from build123d import *

# Parameters (mm, degrees)
SKETCH_1_R           = 1.5
EXTRUDE_1_DEPTH      = 2.5
EXTRUDE_2_DEPTH      = 7
EXTRUDE_2_DEPTH_BACK = 2.5
SKETCH_2_R           = 1.45
SKETCH_2_W           = 22.5
SKETCH_2_H           = 12
SKETCH_3_W           = 8
SKETCH_3_H           = 20
SKETCH_3_R           = 1.5
EXTRUDE_3_DEPTH      = 3
SKETCH_4_R           = 1.5
CUT_EXTRUDE_1_DEPTH  = 54.969899018
SKETCH_6_R           = 3.49128416
EXTRUDE_4_DEPTH      = 2.5
SKETCH_7_R           = 6
CUT_EXTRUDE_3_DEPTH  = 1.5
CUT_EXTRUDE_4_DEPTH  = 1.5
SKETCH_9_R           = 2.5
CUT_EXTRUDE_5_DEPTH  = 1.5
CUT_EXTRUDE_6_DEPTH  = 55.522930956
CHAMFER_1_SIZE       = 2
SKETCH_11_R          = 1.5
CUT_EXTRUDE_8_DEPTH  = 52.232314022
EXTRUDE_START        = -3
EXTRUDE_7_DEPTH      = 3
SKETCH_18_W          = 3
SKETCH_18_H          = 6.085719459
EXTRUDE_9_DEPTH      = 45
SKETCH_19_R          = 1.410967792
SKETCH_19_R_2        = 1.436695047
CUT_EXTRUDE_9_DEPTH  = 45
EXTRUDE_10_DEPTH     = 17.5
SKETCH_21_R          = 1.436695047
SKETCH_21_R_2        = 1.410967792
CUT_EXTRUDE_10_DEPTH = 17.5


with BuildPart() as part:
    # 草图1 → 凸台-拉伸1 (new body)
    with BuildSketch(Plane.XY):
        Polygon((4, 0), (0, 4), (0, 12), (-10, 17), (-10, 27), (45.5, 27), (45.5, 17), (35.5, 12), (35.5, 4), (31.5, 0), align=None)
        with Locations((4, 4)):
            Circle(SKETCH_1_R, mode=Mode.SUBTRACT)
        with Locations((31.5, 4)):
            Circle(SKETCH_1_R, mode=Mode.SUBTRACT)
        with Locations((7, 21)):
            Circle(SKETCH_1_R, mode=Mode.SUBTRACT)
        with Locations((28.5, 21)):
            Circle(SKETCH_1_R, mode=Mode.SUBTRACT)
    extrude(amount=EXTRUDE_1_DEPTH)

    # 草图2 → 凸台-拉伸2 (add, two sides: drawn at the far end of the back side and taken through both)
    with BuildSketch(Plane(origin=(0, 0, 0), x_dir=(-1, 0, 0), z_dir=(0, 0, -1)).offset(-EXTRUDE_2_DEPTH_BACK)):
        with BuildLine():
            Line((-35.2, 28.5), (-9.7, 28.5))
            Line((-9.7, 28.5), (-9.7, 23))
            Line((-9.7, 23), (-8.2, 23))
            Line((-8.2, 23), (-8.2, 22.240967365))
            ThreePointArc((-8.2, 22.240967365), (-10.4, 21), (-8.2, 19.759032635))
            Line((-8.2, 19.759032635), (-8.2, 19))
            Line((-8.2, 19), (-9.7, 19))
            Line((-9.7, 19), (-9.7, 13.5))
            Line((-9.7, 13.5), (-35.2, 13.5))
            Line((-35.2, 13.5), (-35.2, 19))
            Line((-35.2, 19), (-38.2, 19))
            Line((-38.2, 19), (-38.2, 23))
            Line((-38.2, 23), (-35.2, 23))
            Line((-35.2, 23), (-35.2, 28.5))
        make_face()
        with Locations((-35.95, 21)):
            Circle(SKETCH_2_R, mode=Mode.SUBTRACT)
        with Locations((-22.45, 21)):
            Rectangle(SKETCH_2_W, SKETCH_2_H, mode=Mode.SUBTRACT)
    extrude(amount=EXTRUDE_2_DEPTH + EXTRUDE_2_DEPTH_BACK)

    # 草图3 → 凸台-拉伸3 (add)
    with BuildSketch(Plane(origin=(0, 0, 0), x_dir=(-1, 0, 0), z_dir=(0, 0, -1))):
        with Locations((-4, 17)):
            Rectangle(SKETCH_3_W, SKETCH_3_H)
        with Locations((-2.5, 9.5)):
            Circle(SKETCH_3_R, mode=Mode.SUBTRACT)
        with Locations((-2.5, 18.5)):
            Circle(SKETCH_3_R, mode=Mode.SUBTRACT)
    extrude(amount=EXTRUDE_3_DEPTH)

    # 草图4 → 切除-拉伸1 (cut, through all)
    with BuildSketch(Plane(origin=(0, 0, -3), x_dir=(-1, 0, 0), z_dir=(0, 0, -1))):
        with Locations((-2.5, 9.5)):
            Circle(SKETCH_4_R)
        with Locations(Location((-7, 21, 0), (0, 0, 228.189685104))):
            Circle(SKETCH_4_R)
    extrude(amount=-CUT_EXTRUDE_1_DEPTH, mode=Mode.SUBTRACT)

    # 草图6 → 凸台-拉伸4 (add)
    with BuildSketch(Plane(origin=(0, 0, 0), x_dir=(-1, 0, 0), z_dir=(0, 0, -1))):
        with Locations((-27, 21)):
            Circle(SKETCH_6_R)
    extrude(amount=-EXTRUDE_4_DEPTH)

    # 草图7 → 切除-拉伸3 (cut)
    with BuildSketch(Plane(origin=(0, 0, 0), x_dir=(-1, 0, 0), z_dir=(0, 0, -1))):
        with Locations((-27.7, 21)):
            Circle(SKETCH_7_R)
    extrude(amount=-CUT_EXTRUDE_3_DEPTH, mode=Mode.SUBTRACT)

    # 草图8 → 切除-拉伸4 (cut)
    with BuildSketch(Plane(origin=(0, 0, 0), x_dir=(-1, 0, 0), z_dir=(0, 0, -1))):
        with BuildLine():
            ThreePointArc((-21.71878059, 17.962224138), (-18.800764933, 20.795559838), (-21.585591732, 23.759905678))
            ThreePointArc((-21.585591732, 23.759905678), (-22.24975442, 23.944667862), (-22.761132033, 24.406990344))
            ThreePointArc((-22.761132033, 24.406990344), (-21.701582619, 20.862199682), (-22.92279575, 17.369804474))
            ThreePointArc((-22.92279575, 17.369804474), (-22.39072715, 17.808156096), (-21.71878059, 17.962224138))
        make_face()
    extrude(amount=-CUT_EXTRUDE_4_DEPTH, mode=Mode.SUBTRACT)

    # 草图9 → 切除-拉伸5 (cut)
    with BuildSketch(Plane(origin=(0, 0, 1.5), x_dir=(-1, 0, 0), z_dir=(0, 0, -1))):
        with Locations((-27.7, 21)):
            Circle(SKETCH_9_R)
    extrude(amount=-CUT_EXTRUDE_5_DEPTH, mode=Mode.SUBTRACT)

    # 草图10 → 切除-拉伸6 (cut, through all)
    with BuildSketch(Plane.XY.offset(2.5)):
        Polygon((-6, 27), (-6, 15), (-10, 17), (-10, 27), align=None)
        Polygon((41.5, 27), (41.5, 15), (45.5, 17), (45.5, 27), align=None)
    extrude(amount=-CUT_EXTRUDE_6_DEPTH, mode=Mode.SUBTRACT)

    # 倒角1
    chamfer_1_edges = [part.edges().sort_by_distance(p)[0] for p in [
        (-6, 27, 1.25),
        (41.5, 27, 1.25),
    ]]
    chamfer(chamfer_1_edges, length=CHAMFER_1_SIZE)

    # 草图11 → 切除-拉伸8 (cut, through all)
    with BuildSketch(Plane.XY.offset(2.5)):
        with Locations((6, 21)):
            Circle(SKETCH_11_R)
        with Locations((7, 21)):
            Circle(SKETCH_11_R)
    extrude(amount=-CUT_EXTRUDE_8_DEPTH, mode=Mode.SUBTRACT)

    # 草图12 → 凸台-拉伸7 (add)
    with BuildSketch(Plane.XY.offset(2.5).offset(EXTRUDE_START)):
        with BuildLine():
            ThreePointArc((6.5, 19.585786438), (8.5, 21), (6.5, 22.414213562))
            ThreePointArc((6.5, 22.414213562), (7.5, 21), (6.5, 19.585786438))
        make_face()
    extrude(amount=EXTRUDE_7_DEPTH)

    # 草图18 → 凸台-拉伸9 (add)
    with BuildSketch(Plane(origin=(8, 0, 0), x_dir=(0, 0, -1), z_dir=(1, 0, 0))):
        with Locations((1.5, 10.04285973)):
            Rectangle(SKETCH_18_W, SKETCH_18_H)
    extrude(amount=EXTRUDE_9_DEPTH)

    # 草图19 → 切除-拉伸9 (cut)
    with BuildSketch(Plane(origin=(0, 0, -3), x_dir=(-1, 0, 0), z_dir=(0, 0, -1))):
        with Locations((-42.5, 10.017096625)):
            Circle(SKETCH_19_R)
        with Locations((-48.5, 10.017096625)):
            Circle(SKETCH_19_R_2)
    extrude(amount=-CUT_EXTRUDE_9_DEPTH, mode=Mode.SUBTRACT)

    # 草图20 → 凸台-拉伸10 (add)
    with BuildSketch(Plane(origin=(35.5, 0, 0), x_dir=(0, 0, -1), z_dir=(1, 0, 0))):
        Polygon((-2.5, 15), (-2.5, 12), (-2.5, 4), (0, 4), (0, 7), (0, 12), (0, 15), align=None)
    extrude(amount=EXTRUDE_10_DEPTH)

    # 草图21 → 切除-拉伸10 (cut)
    with BuildSketch(Plane(origin=(0, 0, 0), x_dir=(-1, 0, 0), z_dir=(0, 0, -1))):
        with Locations((-48.5, 10.017096625)):
            Circle(SKETCH_21_R)
        with Locations((-42.5, 10.017096625)):
            Circle(SKETCH_21_R_2)
    extrude(amount=-CUT_EXTRUDE_10_DEPTH, mode=Mode.SUBTRACT)


solid = part.part
Read the model definition and answer for the solid it produces. Units are mm, in the model's axes. A direction names the side the tool comes from. Coordinates: 2 decimals unless noted, no trailing zeros. Order: outer loops, then holes, each group sorted by start corner. A loop starts at its lowest first (then second) coordinate and runs counter-clockwise, first axis right, second up. Notation, with made-up numbers: (-40, 24.5) - (6, 24.5) arc R12 ccw to (6, 32.5) - close; hole circle Ø9 at (37, -39.75). An arc over 180 degrees is marked (long way). Use one line per item in the form item = value.
(1) Section A-A, the plane z = -5 is taken. Give the vertices of the cut face in (x, y), then the cut area to 3 significant figures.
Computed values:
outline = (8.2, 19) - (9.7, 19) - (9.7, 13.5) - (35.2, 13.5) - (35.2, 19) - (38.2, 19) - (38.2, 23) - (35.2, 23) - (35.2, 28.5) - (9.7, 28.5) - (9.7, 23) - (8.2, 23) - (8.2, 22.24) arc R1.45 cw (long way) to (8.2, 19.76) - close; hole (11.2, 15) - (33.7, 15) - (33.7, 27) - (11.2, 27) - close; hole circle Ø2.9 at (35.95, 21)
area = 119 mm²
(2) Straight lines are drawn through the part: L1, parallel to Y at x = 2.5, z = -0.9; L2, parallel to Y at x = 14, z = -1.25; L3, parallel to X at y = 24, z = -5.25. For each, find the intervals that lie inside material, in ascending order.
Computed values:
L1 = 7 to 8, 11 to 17, 20 to 27
L2 = 7 to 13.09, 13.5 to 15, 27 to 28.5
L3 = 9.7 to 11.2, 33.7 to 35.2
(3) Given pin 1 Ø0.6 at (x, y) = (8, 21.5) entering from -Z; pin 2 Ø11 at (x, y) = (27.7, 21) entering from -Z; pin 3 Ø3.5 at (x, y) = (8.95, 21) entering from -Z; pin 4 Ø4.5 at (y, z) = (26.5, -3) entering from +X, each flat-ended and moving along its own axis, determine where each tip first touches the part or whether it passes through.
Computed values:
pin_1 = -0.5
pin_2 = 1.5
pin_3 = -7
pin_4 = 35.2
(4) Section D-D, the plane x = 13 is taken. Give the vertices of the cut face in (y, z), then the cut area to 3 significant figures.
Computed values:
outline = (0, 0) - (7, 0) - (7, -3) - (13.09, -3) - (13.09, 0) - (13.5, 0) - (13.5, -7) - (15, -7) - (15, 0) - (27, 0) - (27, -7) - (28.5, -7) - (28.5, 2.5) - (0, 2.5) - close
area = 111 mm²
(5) Section C-C, the plane z = -2 is taken. Give the number of separate pieces and of enclosed holes in the cut face, then the cut area to 3 significant figures.
Computed values:
separate_pieces = 2
enclosed_holes = 6
area = 516 mm²
(6) Which of the six approach directions +Z, -Z, +X, -X, +Y, -Y give full straight-line access (tool end or side, diameter ignored) to faces 1 (the face through (7.28, 22.474, -1.768)), 2 (the face through (20, 4, 0)), 3 (the face through (37, 19, -3)), 4 (the face through (37, 27, 1)), 5 (the face through (3, 27, 0))?
Computed values:
face_1 = -Z
face_2 = -Z, +X, -X, -Y
face_3 = -Z, +X
face_4 = +Z, -Z, +X, +Y
face_5 = +Z, -Z, -X, +Y
(7) Section B-B, the plane x = 48.5 is taken. Give the vertices of the cut face in (y, z).
Computed values:
outline = (4, 0) - (7, 0) - (7, -3) - (8.58, -3) - (8.58, 2.5) - (4, 2.5) - close; (11.45, -3) - (13.09, -3) - (13.09, 0) - (15, 0) - (15, 2.5) - (11.45, 2.5) - close
